Work out the finished part from the listing and answer in its coordinate system (mm). A direction names the side the tool comes from. Round coordinates to 2 decimals unless told otherwise and drop trailing zeros. Loops run counter-clockwise (first coordinate to the right, second up) from the corner with the lowest first, then second, coordinate; pieces in that order, holes last. Notation, with made-up numbers: (8.5, 67) - (12.5, 67) arc R8 cw to (12.5, 72) - close; hole circle Ø9 at (55, 25). An arc over 180 degrees is marked (long way). Answer as CSV lines item,"result". Start each with the question number.
Q1. The mould has two halves that part along X. Classify faces 3 (the face through (40.444, -3, -2)), 4 (the face through (17, -31.277, -2)), 5 (the face through (-71.556, -2, -2)): +X half, -X half, draft (parallel to the pull), parting line (faces both ways), or undercut.
Q2. Section A-A on x = 66.5 is taken. Write down the section's boundary in (y, z).
Q3. Straight lines are drawn through the part: L1, parallel to X at y = -12.5, z = -1.3; L2, parallel to Y at x = 62, z = -2.4; L3, parallel to X at y = -3, z = -0.95. For each, find the intervals that lie inside material, in ascending order. Write a range as [from, to].
Q4. For faces 1 (the face through (-25, -12.777, -2)), 2 (the face through (17, -2, 0)), determine the directions among +Z, -Z, +X, -X, +Y, -Y from which every point of the face is accessible in a straight line to the end or side of a thin tool.
Q5. Section B-B on z = -2 is taken. Count the separate pieces of the cut face and the enclosed holes in it, then the cut area to 3 significant figures.
```python
from build123d import *

# Parameters (mm, degrees)
SKETCH1_R           = 1.5
SKETCH1_W           = 43
SKETCH1_H           = 20
BOSS_EXTRUDE3_DEPTH = 4


with BuildPart() as part:
    # Sketch1 → Boss-Extrude3 (new body)
    with BuildSketch(Plane.XY):
        Polygon((8.44359092, 25.723284589), (-71.55640908, 25.723284589), (-71.55640908, -31.276715411), (8.44359092, -31.276715411), (28.44359092, -31.276715411), (108.44359092, -31.276715411), (108.44359092, 25.723284589), (28.44359092, 25.723284589), align=None)
        with Locations((-48.05640908, -23.776715411)):
            Circle(SKETCH1_R, mode=Mode.SUBTRACT)
        with Locations((-8.05640908, -23.776715411)):
            Circle(SKETCH1_R, mode=Mode.SUBTRACT)
        with Locations((-61.55640908, -2.776715411)):
            Circle(SKETCH1_R, mode=Mode.SUBTRACT)
        with Locations((-25.05640908, -2.776715411)):
            Rectangle(SKETCH1_W, SKETCH1_H, mode=Mode.SUBTRACT)
        with Locations((44.94359092, -23.776715411)):
            Circle(SKETCH1_R, mode=Mode.SUBTRACT)
        with Locations((84.94359092, -23.776715411)):
            Circle(SKETCH1_R, mode=Mode.SUBTRACT)
        with Locations((61.94359092, -2.776715411)):
            Rectangle(SKETCH1_W, SKETCH1_H, mode=Mode.SUBTRACT)
        with Locations((98.44359092, -2.776715411)):
            Circle(SKETCH1_R, mode=Mode.SUBTRACT)
        with Locations((-48.05640908, 18.223284589)):
            Circle(SKETCH1_R, mode=Mode.SUBTRACT)
        with Locations((-8.05640908, 18.223284589)):
            Circle(SKETCH1_R, mode=Mode.SUBTRACT)
        with Locations((44.94359092, 18.223284589)):
            Circle(SKETCH1_R, mode=Mode.SUBTRACT)
        with Locations((84.94359092, 18.223284589)):
            Circle(SKETCH1_R, mode=Mode.SUBTRACT)
    extrude(amount=-BOSS_EXTRUDE3_DEPTH)


solid = part.part
```
Findings:
1,face 3,"undercut"
1,face 4,"draft"
1,face 5,"-X half"
2,outline,"(-31.28, -4) - (-12.78, -4) - (-12.78, 0) - (-31.28, 0) - close; (7.22, -4) - (25.72, -4) - (25.72, 0) - (7.22, 0) - close"
3,L1,"x = [-71.56, -46.56], [-3.56, 40.44], [83.44, 108.44]"
3,L2,"y = [-31.28, -12.78], [7.22, 25.72]"
3,L3,"x = [-71.56, -63.04], [-60.07, -46.56], [-3.56, 40.44], [83.44, 96.96], [99.93, 108.44]"
4,face 1,"+Z, -Z"
4,face 2,"+Z, +X, -X, +Y, -Y"
5,separate pieces,"1"
5,enclosed holes,"12"
5,area,"8,470 mm^2"
